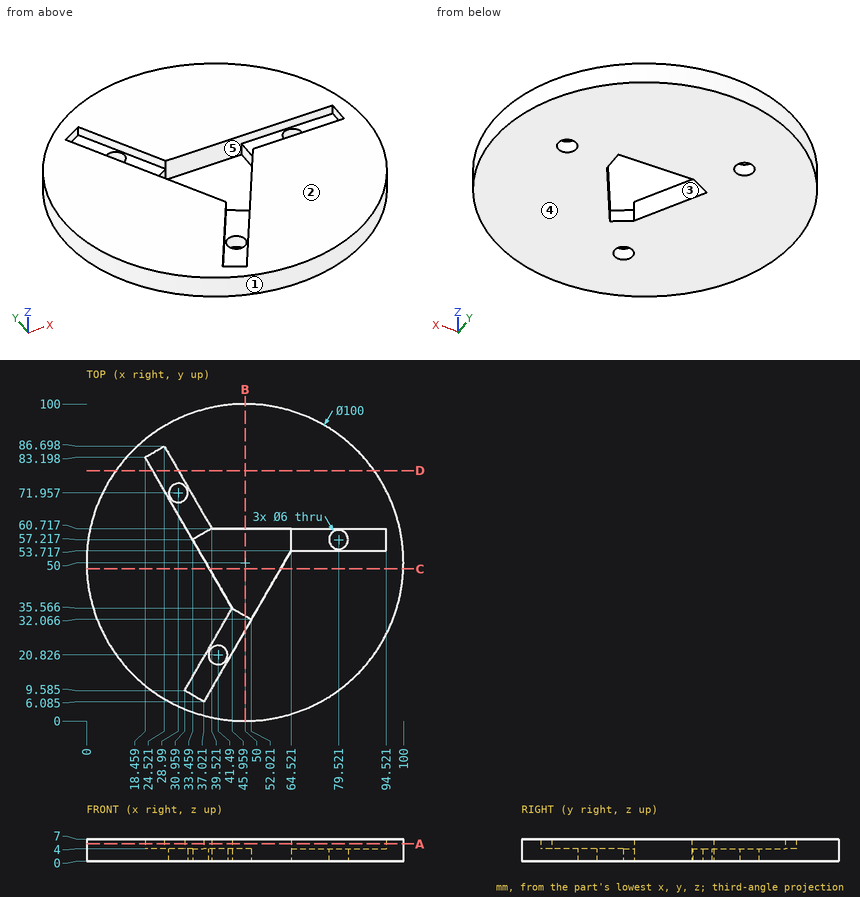
Geometry: see drawing. Coordinates: mm, zero at the bounding-box minimum. A direction names the side the tool comes from. Give positions to 0.01 mm unless a question says otherwise; leave off trailing zeros. Loops run counter-clockwise (first coordinate to the right, second up) from the corner with the lowest first, then second, coordinate; pieces in that order, holes last. Notation, with made-up numbers: (36.25, -1.75) -> (45.25, -1.75) arc R30 cw to (45.25, 22.25) -> close; hole circle Ø4 at (-7.75, 12.25). An arc over 180 degrees is marked (long way). Use CSV: the item, a comma, the result in double quotes.
(1) Cut plane D-D (y = 79). Output: boundary loops of the cut face in (x, z) (1 decimal).
From the geometry:
outline,"(9.3, 0) -> (90.7, 0) -> (90.7, 7) -> (29, 7) -> (29, 4) -> (20.9, 4) -> (20.9, 7) -> (9.3, 7) -> close"
(2) Ray query, line 1 along X through (y, z) = (32.5, 3.5) (1 decimal); line 2 along Z through (x, y) = (34, 60.5); line 3 along Y through (x, z) = (40.5, 1.5) (1 decimal). Return the intervals inside material, ascending. Write a range as [from, to].
From the geometry:
line 1,"[3.2, 51.3], [52.3, 96.8]"
line 2,"[0, 4]"
line 3,"[0.9, 18], [23.7, 45], [60.7, 99.1]"
(3) First-contact query: P1, Ø5.5, axis at x = 28.99, y = 71.96, coming from the -Z side; P2, Ø1.5, axis at x = 86.5, z = 5.5, coming from the +Y side (1 decimal); P3, Ø1.5, axis at y = 58, z = 6, coming from the -X side; P4, Ø9.5, axis at x = 79.52, y = 57.22, coming from the -Z side. Flat tips, straight axial feed; report the tip coordinate or a pass-through.
From the geometry:
P1,"through"
P2,"y = 85"
P3,"x = 0.53"
P4,"z = 0"
(4) Cut plane B-B (x = 50). Output: boundary loops of the cut face in (y, z).
From the geometry:
outline,"(0, 0) -> (33.23, 0) -> (33.23, 4) -> (28.57, 4) -> (28.57, 7) -> (0, 7) -> close; (60.72, 0) -> (100, 0) -> (100, 7) -> (60.72, 7) -> close"
(5) Cut plane A-A (z = 5.5). Output: boundary loops of the cut face in (x, y) (1 decimal).
From the geometry:
outline,"circle Ø100 at (50, 50); hole (18.5, 83.2) -> (46, 35.6) -> (31, 9.6) -> (37, 6.1) -> (64.5, 53.7) -> (94.5, 53.7) -> (94.5, 60.7) -> (39.5, 60.7) -> (24.5, 86.7) -> close"
(6) Access query for the marked faces 4 and 5. Directions: +Z, -Z, +X, -X, +Y, -Y. A direction counts if a zero-diameter tool reaches every point of the face in a straight line with its end or side. Return the directions, or none.
From the geometry:
face 4,"-Z, +X, -X, +Y, -Y"
face 5,"+Z"
(7) Cut plane C-C (y = 48). Output: boundary loops of the cut face in (x, z).
From the geometry:
outline,"(0.04, 0) -> (38.78, 0) -> (38.78, 7) -> (0.04, 7) -> close; (61.22, 0) -> (99.96, 0) -> (99.96, 7) -> (61.22, 7) -> close"
(8) Pull-direction query (X, two-part tool) for the marked faces 1, 2 and 3; classes: released by +X, released by -X, zero draft, split by the parting line, or undercut.
From the geometry:
face 1,"split by the parting line"
face 2,"zero draft"
face 3,"undercut"
